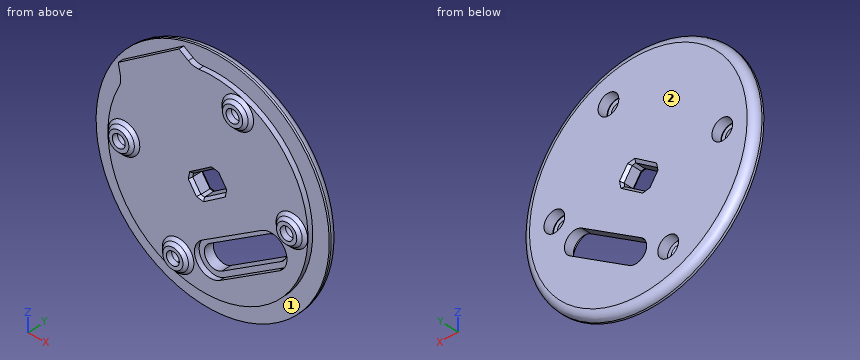
from build123d import *
from build123d.topology import SkipClean

# Parameters (mm, degrees)
SKETCH1_R           = 22.5
BOSS_EXTRUDE1_DEPTH = 1.9
SKETCH2_R           = 1.25
CUT_EXTRUDE1_DEPTH  = 32.876480358
CUT_EXTRUDE2_DEPTH  = 3
SKETCH5_R           = 2
BOSS_EXTRUDE2_DEPTH = 1
SKETCH6_R           = 2
CUT_EXTRUDE3_DEPTH  = 2
FILLET2_R           = 1.5
SKETCH7_R           = 2.5
SKETCH7_R_2         = 1.25
BOSS_EXTRUDE3_DEPTH = 1.1
CHAMFER2_SIZE       = 0.55
BOSS_EXTRUDE4_START = 0.9
SKETCH10_R          = 2
SKETCH10_R_2        = 1.25
BOSS_EXTRUDE4_DEPTH = 0.9
CUT_EXTRUDE4_DEPTH  = 33.070235422
CHAMFER3_SIZE       = 0.5


with BuildPart() as part:
    # Sketch1 → Boss-Extrude1 (new body)
    with BuildSketch(Plane(origin=(0, 0, 0), x_dir=(1, 0, 0), z_dir=(0, 1, 0))):
        with Locations(Location((0, 0, 0), (0, 0, 90))):
            Circle(SKETCH1_R)
    extrude(amount=BOSS_EXTRUDE1_DEPTH)

    # Sketch2 → Cut-Extrude1 (cut, through all)
    with BuildSketch(Plane.XZ):
        with Locations(Location((16.199395554, -0.312653275, 0), (0, 0, 270))):
            Circle(SKETCH2_R)
        with Locations(Location((-5.762032101, -15.143217553, 0), (0, 0, 270))):
            Circle(SKETCH2_R)
        with Locations(Location((-16.199392803, 0.312657063, 0), (0, 0, 270))):
            Circle(SKETCH2_R)
        with Locations(Location((5.762036646, 15.143220658, 0), (0, 0, 270))):
            Circle(SKETCH2_R)
    extrude(amount=-CUT_EXTRUDE1_DEPTH, mode=Mode.SUBTRACT)

    # Sketch3 → Cut-Extrude2 (cut)
    with BuildSketch(Plane(origin=(0, 1.9, 0), x_dir=(1, 0, 0), z_dir=(0, 1, 0))):
        with BuildLine():
            Line((-0.566479918, 11.117262385), (10.889757234, 3.975509775))
            ThreePointArc((10.889757234, 3.975509775), (13.92054075, 4.67861096), (13.217439566, 7.709394476))
            Line((13.217439566, 7.709394476), (1.761202414, 14.851147086))
            ThreePointArc((1.761202414, 14.851147086), (-1.269581102, 14.148045901), (-0.566479918, 11.117262385))
        make_face()
    extrude(amount=-CUT_EXTRUDE2_DEPTH, mode=Mode.SUBTRACT)

    # Sketch5 → Boss-Extrude2 (add)
    with BuildSketch(Plane.XZ):
        with BuildLine():
            ThreePointArc((-17.179194793, 8.795752741), (-16.857328224, 9.81864057), (-16.891461695, 10.890429965))
            Line((-16.891461695, 10.890429965), (-17.314006113, 12.972955453))
            Line((-17.314006113, 12.972955453), (-5.575167705, 20.900200554))
            Line((-5.575167705, 20.900200554), (-3.772911963, 19.726806718))
            ThreePointArc((-3.772911963, 19.726806718), (-2.798329578, 19.30288327), (-1.738658435, 19.221526132))
            ThreePointArc((-1.738658435, 19.221526132), (10.800253719, -15.9951405), (-17.179194793, 8.795752741))
        make_face()
        with Locations(Location((-5.762032101, -15.143217553, 0), (0, 0, 270))):
            Circle(SKETCH5_R, mode=Mode.SUBTRACT)
        with Locations(Location((16.199395554, -0.312653275, 0), (0, 0, 270))):
            Circle(SKETCH5_R, mode=Mode.SUBTRACT)
        with Locations(Location((5.762036647, 15.143220658, 0), (0, 0, 270))):
            Circle(SKETCH5_R, mode=Mode.SUBTRACT)
        with Locations(Location((-16.199392803, 0.312657063, 0), (0, 0, 270))):
            Circle(SKETCH5_R, mode=Mode.SUBTRACT)
        with BuildLine():
            ThreePointArc((-1.095498629, -10.268652225), (-2.118191262, -14.677064613), (2.290221126, -15.699757245))
            Line((2.290221126, -15.699757245), (13.746458277, -8.558004636))
            ThreePointArc((13.746458277, -8.558004636), (14.76915091, -4.149592248), (10.360738522, -3.126899616))
            Line((10.360738522, -3.126899616), (-1.095498629, -10.268652225))
        make_face(mode=Mode.SUBTRACT)
    extrude(amount=BOSS_EXTRUDE2_DEPTH)

    # Sketch6 → Cut-Extrude3 (cut)
    with SkipClean():  # the faces are left unmerged after this step: merging them gives an invalid solid
        with BuildSketch(Plane(origin=(0, 1.9, 0), x_dir=(1, 0, 0), z_dir=(0, 1, 0))):
            with Locations(Location((-16.199392803, -0.312657063, 0), (0, 0, 270))):
                Circle(SKETCH6_R)
            with Locations(Location((-5.762030762, 15.143217579, 0), (0, 0, 270))):
                Circle(SKETCH6_R)
            with Locations(Location((5.762036646, -15.143220658, 0), (0, 0, 270.000000006))):
                Circle(SKETCH6_R)
            with Locations(Location((16.199395554, 0.312653275, 0), (0, 0, 270))):
                Circle(SKETCH6_R)
        extrude(amount=-CUT_EXTRUDE3_DEPTH, mode=Mode.SUBTRACT)
    add(part.part.scale(1), mode=Mode.REPLACE)  # the faces are merged on a copy

    # Fillet2
    fillet2_edges = [part.edges().sort_by_distance(p)[0] for p in [
        (0, 1.9, 22.5),
    ]]
    fillet(fillet2_edges, radius=FILLET2_R)

    # Sketch7 → Boss-Extrude3 (add)
    # profile 1 of 4: a face of its own
    with BuildSketch(Plane.XZ.offset(1)):
        with Locations(Location((-16.199392803, 0.312657063, 0), (0, 0, 270))):
            Circle(SKETCH7_R)
        with Locations(Location((-16.199392803, 0.312657063, 0), (0, 0, 270))):
            Circle(SKETCH7_R_2, mode=Mode.SUBTRACT)
    # profile 2 of 4: a face of its own
    with BuildSketch(Plane.XZ.offset(1)):
        with Locations(Location((5.762036647, 15.143220658, 0), (0, 0, 270))):
            Circle(SKETCH7_R)
        with Locations(Location((5.762036647, 15.143220658, 0), (0, 0, 270))):
            Circle(SKETCH7_R_2, mode=Mode.SUBTRACT)
    # profile 3 of 4: a face of its own
    with BuildSketch(Plane.XZ.offset(1)):
        with Locations(Location((16.199395554, -0.312653275, 0), (0, 0, 270))):
            Circle(SKETCH7_R)
        with Locations(Location((16.199395554, -0.312653275, 0), (0, 0, 270))):
            Circle(SKETCH7_R_2, mode=Mode.SUBTRACT)
    # profile 4 of 4: a face of its own
    with BuildSketch(Plane.XZ.offset(1)):
        with Locations(Location((-5.762032101, -15.143217553, 0), (0, 0, 270))):
            Circle(SKETCH7_R)
        with Locations(Location((-5.762032101, -15.143217553, 0), (0, 0, 270))):
            Circle(SKETCH7_R_2, mode=Mode.SUBTRACT)
    extrude(amount=BOSS_EXTRUDE3_DEPTH)

    # Chamfer2
    chamfer2_edges = [part.edges().sort_by_distance(p)[0] for p in [
        (-16.199392803, -2.1, 2.812657063),
        (-16.199392803, -1, 2.812657063),
        (5.762036647, -2.1, 17.643220658),
        (5.762036647, -1, 17.643220658),
        (16.199395554, -2.1, 2.187346725),
        (16.199395554, -1, 2.187346725),
        (-5.762032101, -2.1, -12.643217553),
        (-5.762032101, -1, -12.643217553),
    ]]
    chamfer(chamfer2_edges, length=CHAMFER2_SIZE - 0.0001)  # a hair under: the kernel refuses the full size

    # Sketch10 → Boss-Extrude4 (add)
    # profile 1 of 4: a face of its own
    with BuildSketch(Plane(origin=(0, -1, 0), x_dir=(1, 0, 0), z_dir=(0, 1, 0)).offset(BOSS_EXTRUDE4_START)):
        with Locations(Location((-5.762032101, 15.143217553, 0), (0, 0, 270))):
            Circle(SKETCH10_R)
        with Locations(Location((-5.762032101, 15.143217553, 0), (0, 0, 270))):
            Circle(SKETCH10_R_2, mode=Mode.SUBTRACT)
    # profile 2 of 4: a face of its own
    with BuildSketch(Plane(origin=(0, -1, 0), x_dir=(1, 0, 0), z_dir=(0, 1, 0)).offset(BOSS_EXTRUDE4_START)):
        with Locations(Location((5.762036647, -15.143220658, 0), (0, 0, 270))):
            Circle(SKETCH10_R)
        with Locations(Location((5.762036647, -15.143220658, 0), (0, 0, 270))):
            Circle(SKETCH10_R_2, mode=Mode.SUBTRACT)
    # profile 3 of 4: a face of its own
    with BuildSketch(Plane(origin=(0, -1, 0), x_dir=(1, 0, 0), z_dir=(0, 1, 0)).offset(BOSS_EXTRUDE4_START)):
        with Locations(Location((16.199395554, 0.312653275, 0), (0, 0, 270))):
            Circle(SKETCH10_R)
        with Locations(Location((16.199395554, 0.312653275, 0), (0, 0, 270))):
            Circle(SKETCH10_R_2, mode=Mode.SUBTRACT)
    # profile 4 of 4: a face of its own
    with BuildSketch(Plane(origin=(0, -1, 0), x_dir=(1, 0, 0), z_dir=(0, 1, 0)).offset(BOSS_EXTRUDE4_START)):
        with Locations(Location((-16.199392803, -0.312657063, 0), (0, 0, 270))):
            Circle(SKETCH10_R)
        with Locations(Location((-16.199392803, -0.312657063, 0), (0, 0, 270))):
            Circle(SKETCH10_R_2, mode=Mode.SUBTRACT)
    extrude(amount=-BOSS_EXTRUDE4_DEPTH)

    # Sketch11 → Cut-Extrude4 (cut, through all)
    with BuildSketch(Plane(origin=(0, 1.9, 0), x_dir=(1, 0, 0), z_dir=(0, 1, 0))):
        Polygon((1.366935798, -3.196360259), (-3.654112636, 0.191121747), (-1.532974971, 3.335148765), (3.488073463, -0.052333241), align=None)
    extrude(amount=-CUT_EXTRUDE4_DEPTH, mode=Mode.SUBTRACT)

    # Chamfer3
    chamfer3_edges = [part.edges().sort_by_distance(p)[0] for p in [
        (0.977549246, -1, -1.641407762),
        (-2.593543803, -1, -1.763135256),
        (-1.143588419, -1, 1.502619256),
        (2.42750463, -1, 1.62434675),
        (3.488073463, 0.45, 0.052333241),
        (1.366935798, 0.45, 3.196360259),
        (-3.654112636, 0.45, -0.191121747),
        (-1.532974971, 0.45, -3.335148765),
        (2.42750463, 1.9, 1.62434675),
        (0.977549246, 1.9, -1.641407762),
        (-2.593543803, 1.9, -1.763135256),
        (-1.143588419, 1.9, 1.502619256),
    ]]
    chamfer(chamfer3_edges, length=CHAMFER3_SIZE)


solid = part.part
Verification items for the finished model (mm, model axes). Face numbers are marked on the shaded views. A direction names the side the tool comes from. Give positions to 0.01 mm unless a question says otherwise; leave off trailing zeros. Use CSV: the item, a comma, the result in double quotes.
1) Material ranges on line 1 along X through (y, z) = (-0.4, 0); line 2 along Z through (x, y) = (7, 0.45); line 3 along Y through (x, z) = (-13.5, 16), recorded low to high.
Final values:
line 1,"-19.3 to -17.41, -14.99 to -3.26, 3.12 to 14.99, 17.41 to 19.3"
line 2,"-21.38 to -11.59, -6.4 to 13.57, 16.71 to 21.38"
line 3,"0 to 1.9"
2) Go/stop test with flat-tipped pins: pin 1 Ø1 at (x, y) = (-2, 1) entering from +Z; pin 2 Ø3 at (x, z) = (5.76, 15.14) entering from +Y; pin 3 Ø3 at (x, z) = (-5.5, 14) entering from -Y; pin 4 Ø2 at (x, z) = (-16.2, 0.31) entering from -Y. Record where each tip stops, or that it passes through.
Final values:
pin 1,"z = 22.42"
pin 2,"y = -0.1"
pin 3,"y = -1"
pin 4,"through"
3) Access from +Z, -Z, +X, -X, +Y, -Y to the whole of each face (thin tool, end or side, straight path). Record for the marked faces 1 and 2.
Final values:
face 1,"-Y"
face 2,"+Z, -Z, +X, -X, +Y"
